```python
from build123d import *

# Parameters (mm, degrees)
SKETCH1_W           = 167.6
SKETCH1_H           = 58.4
BOSS_EXTRUDE1_DEPTH = 2
SKETCH2_R           = 1.6
CUT_EXTRUDE1_DEPTH  = 89.764181965


with BuildPart() as part:
    # Sketch1 → Boss-Extrude1 (new body)
    with BuildSketch(Plane(origin=(0, 0, 0), x_dir=(1, 0, 0), z_dir=(0, 1, 0))):
        Rectangle(SKETCH1_W, SKETCH1_H)
    extrude(amount=BOSS_EXTRUDE1_DEPTH)

    # Sketch2 → Cut-Extrude1 (cut, through all)
    with BuildSketch(Plane(origin=(0, 0, 0), x_dir=(1, 0, 0), z_dir=(0, 1, 0))):
        with Locations(Location((-80, 25.4, 0), (0, 0, 270))):
            Circle(SKETCH2_R)
        with Locations(Location((-80, -25.4, 0), (0, 0, 270))):
            Circle(SKETCH2_R)
        with Locations(Location((80, 25.4, 0), (0, 0, 270))):
            Circle(SKETCH2_R)
        with Locations(Location((80, -25.4, 0), (0, 0, 270))):
            Circle(SKETCH2_R)
    extrude(amount=CUT_EXTRUDE1_DEPTH, mode=Mode.SUBTRACT)


solid = part.part
```
The listing builds one solid part. Answer for the finished solid, in the listing's coordinates (mm). Give positions to 0.01 mm unless a question says otherwise; leave off trailing zeros. Order: outer loops, then holes, each group sorted by start corner. A loop starts at its lowest first (then second) coordinate and runs counter-clockwise, first axis right, second up. Notation, with made-up numbers: (52, 8.5) -> (108, 8.5) arc R9 cw to (108, 12.5) -> close; hole circle Ø1 at (19, -29). An arc over 180 degrees is marked (long way). Answer as CSV lines item,"result". Start each with the question number.
Q1. Given pin 1 (5 mm diameter, centred on x = -80, z = 25.4, fed in from +Y), flat-ended and moving along its own axis, determine where the tip first touches the part or whether it passes through.
Q2. A cutting plane is placed at B-B (z = 25.4). Determine the outline of the cut face in (x, y), then the cut area to 3 significant figures.
Q3. Determine the mould class of faces 1 (the cylindrical face through (-80, 1, 27)), 2 (the flat face through (-1, 0, 0)) for opening direction X: pulls with the +X half, pulls with the -X half, needs draft (parallel to the pull), parting line crosses it, or undercut.
Q4. A cutting plane is placed at A-A (x = 80). Determine the outline of the cut face in (y, z), then the cut area to 3 significant figures.
Q5. Find the intervals of material crossed by L1, parallel to X at y = 1.65, z = -25.4; L2, parallel to Z at x = -80, y = 1.1; L3, parallel to X at y = 1.95, z = 26.5, in increasing order.
Results found:
1,pin 1,"y = 2"
2,outline,"(-83.8, 0) -> (-81.6, 0) -> (-81.6, 2) -> (-83.8, 2) -> close; (-78.4, 0) -> (78.4, 0) -> (78.4, 2) -> (-78.4, 2) -> close; (81.6, 0) -> (83.8, 0) -> (83.8, 2) -> (81.6, 2) -> close"
2,area,"322 mm2"
3,face 1,"undercut"
3,face 2,"needs draft"
4,outline,"(0, -29.2) -> (2, -29.2) -> (2, -27) -> (0, -27) -> close; (0, -23.8) -> (2, -23.8) -> (2, 23.8) -> (0, 23.8) -> close; (0, 27) -> (2, 27) -> (2, 29.2) -> (0, 29.2) -> close"
4,area,"104 mm2"
5,L1,"-83.8 to -81.6, -78.4 to 78.4, 81.6 to 83.8"
5,L2,"-29.2 to -27, -23.8 to 23.8, 27 to 29.2"
5,L3,"-83.8 to -81.16, -78.84 to 78.84, 81.16 to 83.8"
